Here's how the part is built. I have some questions about the finished solid (model axes, mm). Round coordinates to 2 decimals unless told otherwise and drop trailing zeros. Write each loop counter-clockwise with the first axis right and the second up, starting at its lowest first coordinate (ties: lowest second). Pieces come first, ordered by that corner, then holes. Notation, with made-up numbers: (-39.5, 73.25) -> (-32.5, 73.25) arc R32 cw to (-32.5, 103.25) -> close; hole circle Ø9 at (34, -29.5). An arc over 180 degrees is marked (long way). Answer in a Markdown table with one row per item.
from build123d import *

# Parameters (mm, degrees)
SKETCH2_R             = 8.509
BOSS_EXTRUDE1_DEPTH   = 2.25
M2_CLEARANCE_HOLE1_D  = 2.4
CHAMFER1_SIZE         = 0.75
CHAMFER2_SIZE         = 0.75
CHAMFER3_SIZE         = 0.75
M4X0_7_TAPPED_HOLE1_D = 3.3
SKETCH11_R            = 1
CUT_EXTRUDE1_DEPTH    = 4.509


with BuildPart() as part:
    # Sketch2 → Boss-Extrude1 (new body, symmetric)
    with BuildSketch(Plane.XY):
        Circle(SKETCH2_R)
    extrude(amount=BOSS_EXTRUDE1_DEPTH, both=True)

    # M2 Clearance Hole1 (through all)
    with Locations(Plane.XY.offset(2.25)):
        with Locations((-6.223, 0), (3.1115, 5.389276088), (3.1115, -5.389276088)):
            Hole(M2_CLEARANCE_HOLE1_D / 2)

    # Chamfer1
    chamfer1_edges = [part.edges().sort_by_distance(p)[0] for p in [
        (4.3115, -5.389276088, 2.25),
    ]]
    chamfer(chamfer1_edges, length=CHAMFER1_SIZE)

    # Chamfer2
    chamfer2_edges = [part.edges().sort_by_distance(p)[0] for p in [
        (4.3115, 5.389276088, 2.25),
    ]]
    chamfer(chamfer2_edges, length=CHAMFER2_SIZE)

    # Chamfer3
    chamfer3_edges = [part.edges().sort_by_distance(p)[0] for p in [
        (-5.023, 0, 2.25),
    ]]
    chamfer(chamfer3_edges, length=CHAMFER3_SIZE)

    # M4x0.7 Tapped Hole1 (through all)
    with Locations(Plane.XY.offset(2.25)):
        with Locations((0, 0)):
            Hole(M4X0_7_TAPPED_HOLE1_D / 2)

    # Sketch11 → Cut-Extrude1 (cut, through all)
    with BuildSketch(Plane(origin=(5, 0, 0), x_dir=(0, 0, -1), z_dir=(1, 0, 0))):
        Circle(SKETCH11_R)
    extrude(amount=CUT_EXTRUDE1_DEPTH, mode=Mode.SUBTRACT)


solid = part.part
1) We'd pull the mould along Z, two halves only. Please class faces 1 (the face through (5, 0, 0)), 2 (the face through (2.558, -6.454, -0.401)), 3 (the face through (0, -2, -2.25)), 4 (the face through (7, -1, 0)): +Z half, -Z half, draft (parallel to the pull), parting line (faces both ways), or undercut.
Response:
| item | result |
|---|---|
| face 1 | undercut |
| face 2 | draft |
| face 3 | -Z half |
| face 4 | undercut |
2) I want a section at D-D, the plane z = 1.8. List the corners of the cut face in (x, y) for me, and give its area (3 significant figures).
Response:
| item | result |
|---|---|
| outline | circle Ø17.02 at (0, 0); hole circle Ø3 at (-6.22, 0); hole circle Ø3.3 at (0, 0); hole circle Ø3 at (3.11, -5.39); hole circle Ø3 at (3.11, 5.39) |
| area | 198 mm^2 |
3) I want a section at C-C, the plane z = 0.2. List the corners of the cut face in (x, y) for me, and give its area (3 significant figures).
Response:
| item | result |
|---|---|
| outline | (5, -0.98) -> (5, 0.98) -> (8.45, 0.98) arc R8.51 ccw (long way) to (8.45, -0.98) -> close; hole circle Ø2.4 at (-6.22, 0); hole circle Ø3.3 at (0, 0); hole circle Ø2.4 at (3.11, -5.39); hole circle Ø2.4 at (3.11, 5.39) |
| area | 198 mm^2 |
4) I want a section at B-B, the plane x = 0. List the corners of the cut face in (y, z) for me, and give its area (3 significant figures).
Response:
| item | result |
|---|---|
| outline | (-8.51, -2.25) -> (-1.65, -2.25) -> (-1.65, 2.25) -> (-8.51, 2.25) -> close; (1.65, -2.25) -> (8.51, -2.25) -> (8.51, 2.25) -> (1.65, 2.25) -> close |
| area | 61.7 mm^2 |
5) I need wall thicknesses on line 1 (Z direction, x = 6.5, y = 0); line 2 (Y direction, x = 0, z = 0.35); line 3 (Y direction, x = 3.75, z = -0.9). Which ranges of each line are inside material? Lowest first, please. Write a range as [from, to].
Response:
| item | result |
|---|---|
| line 1 | z = [-2.25, -1], [1, 2.25] |
| line 2 | y = [-8.51, -1.65], [1.65, 8.51] |
| line 3 | y = [-7.64, -6.41], [-4.37, 4.37], [6.41, 7.64] |
6) I want a section at A-A, the plane y = 0. List the corners of the cut face in (x, z) for me.
Response:
| item | result |
|---|---|
| outline | (-8.51, -2.25) -> (-7.42, -2.25) -> (-7.42, 1.5) -> (-8.17, 2.25) -> (-8.51, 2.25) -> close; (-5.02, -2.25) -> (-1.65, -2.25) -> (-1.65, 2.25) -> (-4.27, 2.25) -> (-5.02, 1.5) -> close; (1.65, -2.25) -> (8.51, -2.25) -> (8.51, -1) -> (5, -1) -> (5, 1) -> (8.51, 1) -> (8.51, 2.25) -> (1.65, 2.25) -> close |
7) For pin 1 (0.6 mm diameter, centred on y = 0, z = 0.5, fed in from +X); pin 2 (3 mm diameter, centred on x = 0, y = 0, fed in from -Z); pin 3 (1 mm diameter, centred on y = -6, z = -1.5, fed in from -X); pin 4 (2 mm diameter, centred on y = 5, z = 0.5, fed in from +X), each with a flat end and sliding along its axis, tell me the tip position at first contact or that it passes through.
Response:
| item | result |
|---|---|
| pin 1 | stops at x = 5 |
| pin 2 | passes through |
| pin 3 | stops at x = -6.49 |
| pin 4 | stops at x = 7.51 |
